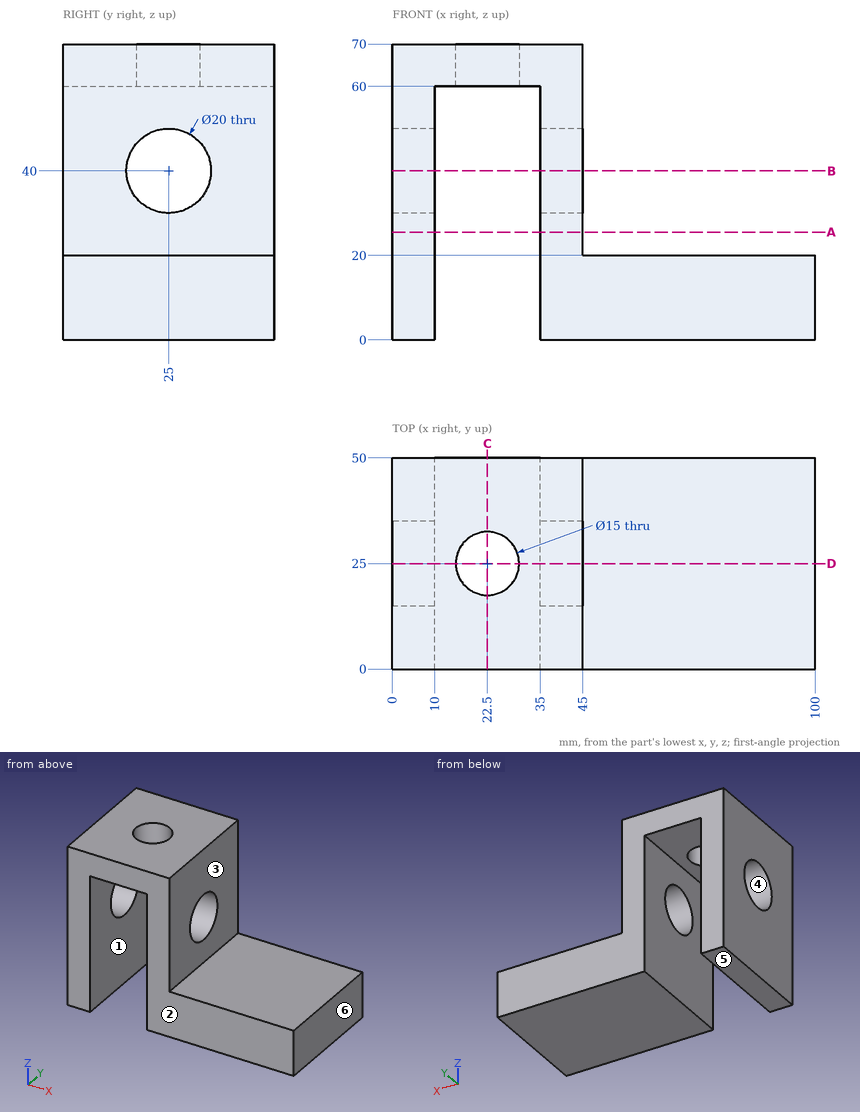
Answer from the drawing. Dimensions are ordinates in mm from the lowest x, y and z of the part. A direction names the side the tool comes from. Coordinates: 2 decimals unless noted, no trailing zeros. Write each loop counter-clockwise with the first axis right and the second up, starting at its lowest first coordinate (ties: lowest second). Pieces come first, ordered by that corner, then holes. Notation, with made-up numbers: M 66,3.25 L 70,3.25 A16 cw 70,9.25 Z; hole C 89,30 d5. An arc over 180 degrees is marked long. Use one line per item in the form item = value. Start each with the question number.
1. The part is cut by section C-C (x = 22.5). Give the vertices of the cut face in (y, z).
2. The part is cut by section D-D (y = 25). Give the vertices of the cut face in (x, z).
3. The part is cut by section A-A (z = 25.5). Give the vertices of the cut face in (x, y), plus the area to 3 significant figures.
4. Each of these flat-tipped pins is pushed along its axis until it touches: P1, Ø4, axis at x = 73.5, y = 16.5, coming from the -Z side; P2, Ø25, axis at x = 86, y = 19, coming from the +Z side; P3, Ø7.5, axis at x = 19.5, y = 34, coming from the -Z side; P4, Ø23, axis at y = 25, z = 40, coming from the +X side. Where does it stop, or does it pass through?
5. A tool of negligible diameter and unlimited length cuts with its end or side. For the marked faces 1, 2 and 3, from which of +Z, -Z, +X, -X, +Y, -Y can it reach the whole face along a straight path? Write none if from no direction.
6. The part is cut by section B-B (z = 40). Give the vertices of the cut face in (x, y), plus the area to 3 significant figures.
7. Straight lines are drawn through the part: probe 1 along X at (y, z) = (45, 4); probe 2 along X at (y, z) = (13.5, 32); probe 3 along Z at (x, y) = (39, 25). For each, find the intervals that lie inside material, in ascending order. Write a range as from..to.
8. The mould has two halves that part along Z. Classify the marked faces 4, 5 and 6: released by +Z, released by -Z, zero draft, split by the parting line, or undercut.
Evaluation:
q1.outline = M 0,60 L 17.5,60 L 17.5,70 L 0,70 Z; M 32.5,60 L 50,60 L 50,70 L 32.5,70 Z
q2.outline = M 0,0 L 10,0 L 10,30 L 0,30 Z; M 0,50 L 10,50 L 10,60 L 15,60 L 15,70 L 0,70 Z; M 30,60 L 35,60 L 35,50 L 45,50 L 45,70 L 30,70 Z; M 35,0 L 100,0 L 100,20 L 45,20 L 45,30 L 35,30 Z
q3.outline = M 0,0 L 10,0 L 10,50 L 0,50 Z; M 35,0 L 45,0 L 45,50 L 35,50 Z
q3.area = 1,000 mm^2
q4.P1 = 0
q4.P2 = 20
q4.P3 = 60
q4.P4 = 45
q5.face_1 = -Z, +Y, -Y
q5.face_2 = +Z, -Z, +X, -X, -Y
q5.face_3 = +Z, +X, +Y, -Y
q6.outline = M 0,0 L 10,0 L 10,15 L 0,15 Z; M 0,35 L 10,35 L 10,50 L 0,50 Z; M 35,0 L 45,0 L 45,15 L 35,15 Z; M 35,35 L 45,35 L 45,50 L 35,50 Z
q6.area = 600 mm^2
q7.probe_1 = 0..10, 35..100
q7.probe_2 = 0..10, 35..45
q7.probe_3 = 0..30, 50..70
q8.face_4 = undercut
q8.face_5 = released by -Z
q8.face_6 = zero draft
